The model under review builds one solid part; all positions refer to its coordinate system, in mm. A direction names the side the tool comes from. Round coordinates to 2 decimals unless told otherwise and drop trailing zeros. Write each loop counter-clockwise with the first axis right and the second up, starting at its lowest first coordinate (ties: lowest second). Pieces come first, ordered by that corner, then holes. Notation, with made-up numbers: (73, 74.5) - (85, 74.5) arc R21 ccw to (85, 95.5) - close; hole circle Ø3 at (69, 10.5). An arc over 180 degrees is marked (long way). Use one line per item in the form item = value.
from build123d import *

# Parameters (mm, degrees)
BOSS_EXTRUDE1_DEPTH = 28
CUT_EXTRUDE1_DEPTH  = 26.5
CUT_EXTRUDE2_DEPTH  = 2.5


with BuildPart() as part:
    # Sketch1 → Boss-Extrude1 (new body)
    with BuildSketch(Plane.XY):
        with BuildLine():
            Line((-20, 26), (20, 26))
            ThreePointArc((20, 26), (22.828427125, 24.828427125), (24, 22))
            Line((24, 22), (24, -22))
            ThreePointArc((24, -22), (22.828427125, -24.828427125), (20, -26))
            Line((20, -26), (-20, -26))
            ThreePointArc((-20, -26), (-22.828427125, -24.828427125), (-24, -22))
            Line((-24, -22), (-24, 22))
            ThreePointArc((-24, 22), (-22.828427125, 24.828427125), (-20, 26))
        make_face()
    extrude(amount=BOSS_EXTRUDE1_DEPTH)

    # Sketch2 → Cut-Extrude1 (cut)
    with BuildSketch(Plane.XY.offset(28)):
        with BuildLine():
            Line((-19.25, 25.25), (19.25, 25.25))
            ThreePointArc((19.25, 25.25), (22.078427125, 24.078427125), (23.25, 21.25))
            Line((23.25, 21.25), (23.25, -21.25))
            ThreePointArc((23.25, -21.25), (22.078427125, -24.078427125), (19.25, -25.25))
            Line((19.25, -25.25), (-19.25, -25.25))
            ThreePointArc((-19.25, -25.25), (-22.078427125, -24.078427125), (-23.25, -21.25))
            Line((-23.25, -21.25), (-23.25, 21.25))
            ThreePointArc((-23.25, 21.25), (-22.078427125, 24.078427125), (-19.25, 25.25))
        make_face()
    extrude(amount=-CUT_EXTRUDE1_DEPTH, mode=Mode.SUBTRACT)

    # Sketch3 → Cut-Extrude2 (cut, through all)
    with BuildSketch(Plane.XY.offset(1.5)):
        with BuildLine():
            Line((-19.5, 9), (-14.5, 9))
            ThreePointArc((-14.5, 9), (-13.792893219, 8.707106781), (-13.5, 8))
            Line((-13.5, 8), (-13.5, -8))
            ThreePointArc((-13.5, -8), (-13.792893219, -8.707106781), (-14.5, -9))
            Line((-14.5, -9), (-19.5, -9))
            ThreePointArc((-19.5, -9), (-20.207106781, -8.707106781), (-20.5, -8))
            Line((-20.5, -8), (-20.5, 8))
            ThreePointArc((-20.5, 8), (-20.207106781, 8.707106781), (-19.5, 9))
        make_face()
    extrude(amount=-CUT_EXTRUDE2_DEPTH, mode=Mode.SUBTRACT)


solid = part.part
(1) To check wall thickness, follow L1, parallel to X at y = 3, z = 15; L2, parallel to Y at x = 6.5, z = 19; L3, parallel to Z at x = 17.5, y = 15. State the ranges of each line that lie inside material, in increasing order.
Geometry results:
L1 = -24 to -23.25, 23.25 to 24
L2 = -26 to -25.25, 25.25 to 26
L3 = 0 to 1.5
(2) The part is to be moulded in two halves that separate along X. For faces 4 (the cylindrical face through (-22.859, 24.797, 13.804)), 5 (the flat face through (0, -26, 14)), 6 (the flat face through (0, 0, 1.5)), say which applies: +X half, -X half, draft (parallel to the pull), parting line (faces both ways), or undercut.
Geometry results:
face_4 = -X half
face_5 = draft
face_6 = undercut
(3) Add section C-C on x = 13. Write out the cut boundary in (y, z), then the cut area to 3 significant figures.
Geometry results:
outline = (-26, 0) - (26, 0) - (26, 28) - (25.25, 28) - (25.25, 1.5) - (-25.25, 1.5) - (-25.25, 28) - (-26, 28) - close
area = 118 mm2
(4) Add section A-A on y = 2. Write out the cut boundary in (x, z).
Geometry results:
outline = (-24, 0) - (-20.5, 0) - (-20.5, 1.5) - (-23.25, 1.5) - (-23.25, 28) - (-24, 28) - close; (-13.5, 0) - (24, 0) - (24, 28) - (23.25, 28) - (23.25, 1.5) - (-13.5, 1.5) - close
(5) Add section B-B on z = 21. Write out the cut boundary in (x, y), then the cut area to 3 significant figures.
Geometry results:
outline = (-24, -22) arc R4 ccw to (-20, -26) - (20, -26) arc R4 ccw to (24, -22) - (24, 22) arc R4 ccw to (20, 26) - (-20, 26) arc R4 ccw to (-24, 22) - close; hole (-23.25, -21.25) arc R4 ccw to (-19.25, -25.25) - (19.25, -25.25) arc R4 ccw to (23.25, -21.25) - (23.25, 21.25) arc R4 ccw to (19.25, 25.25) - (-19.25, 25.25) arc R4 ccw to (-23.25, 21.25) - close
area = 148 mm2
(6) Add section D-D on y = -17. Write out the cut boundary in (x, z).
Geometry results:
outline = (-24, 0) - (24, 0) - (24, 28) - (23.25, 28) - (23.25, 1.5) - (-23.25, 1.5) - (-23.25, 28) - (-24, 28) - close
(7) Insertion check: P1, Ø8, axis at x = 12, y = 20.5, coming from the +Z side. The pin has a flat end and moves straight along its axis. Give the tip position at first contact, or say it passes through.
Geometry results:
P1 = 1.5
(8) Machinability: for faces 1 (the flat face through (-13.5, 0, 1)), 2 (the flat face through (-24, 0, 14)), 3 (the cylindrical face through (-22.047, -24.109, 14.936)), which of the approach directions +Z, -Z, +X, -X, +Y, -Y give a long, thin tool a straight path to every point of the face, cutting with its end or side? Answer none if there is none.
Geometry results:
face_1 = +Z, -Z
face_2 = +Z, -Z, -X, +Y, -Y
face_3 = +Z
